Design review of the part built by this model. Coordinates are the model's own, in mm. Coordinates: 2 decimals unless noted, no trailing zeros. Write each loop counter-clockwise with the first axis right and the second up, starting at its lowest first coordinate (ties: lowest second). Pieces come first, ordered by that corner, then holes.
Q1. Take a section at A-A, the plane x = 0. Write out the cut boundary in (y, z).
Q2. Take a section at B-B, the plane z = 0. Write out the cut boundary in (x, y).
Q3. For L1, parallel to X at y = 1.65, z = 0; L2, parallel to X at y = 0.75, z = -13.5; L3, parallel to X at y = 2.6, z = 2, list the stretches that pass through material, from the lowest coordinate up.
Q4. Take a section at D-D, the plane y = 0.65. State how many separate pieces and enclosed holes the cut face has, plus the area to 3 significant figures.
Q5. Take a section at C-C, the plane x = -18.5. Write out the cut boundary in (y, z), plus the area to 3 significant figures.
Q6. For pin 1 Ø1.5 at (x, y) = (9.5, 0.5) entering from -Z; pin 2 Ø1.5 at (y, z) = (2, -13) entering from -X; pin 3 Ø2.5 at (x, z) = (-9.5, 0) entering from -Y, all flat-tipped, find the tip position at first contact; note any pin that passes through.
from build123d import *

# Parameters (mm, degrees)
SKETCH_1_R      = 25
SKETCH_1_R_2    = 5
SKETCH_1_R_3    = 1.5
SKETCH_1_R_4    = 2.5
EXTRUDE_1_DEPTH = 3


with BuildPart() as part:
    # 草圖1 → 填料-伸長1 (new body)
    with BuildSketch(Plane(origin=(0, 0, 0), x_dir=(1, 0, 0), z_dir=(0, 1, 0))):
        with Locations(Location((0, 0, 0), (0, 0, 270))):
            Circle(SKETCH_1_R)
        with Locations(Location((0, 0, 0), (0, 0, 270))):
            Circle(SKETCH_1_R_2, mode=Mode.SUBTRACT)
        with Locations(Location((-9.5, 0, 0), (0, 0, 270))):
            Circle(SKETCH_1_R_3, mode=Mode.SUBTRACT)
        with Locations(Location((9.5, 0, 0), (0, 0, 270))):
            Circle(SKETCH_1_R_3, mode=Mode.SUBTRACT)
        with Locations(Location((0, 19.5, 0), (0, 0, 270))):
            Circle(SKETCH_1_R_4, mode=Mode.SUBTRACT)
        with Locations(Location((19.5, 0, 0), (0, 0, 270))):
            Circle(SKETCH_1_R_4, mode=Mode.SUBTRACT)
        with Locations(Location((0, -19.5, 0), (0, 0, 270))):
            Circle(SKETCH_1_R_4, mode=Mode.SUBTRACT)
        with Locations(Location((-19.5, 0, 0), (0, 0, 270))):
            Circle(SKETCH_1_R_4, mode=Mode.SUBTRACT)
        with Locations(Location((-13.788582233, 13.788582233, 0), (0, 0, 270))):
            Circle(SKETCH_1_R_3, mode=Mode.SUBTRACT)
        with Locations(Location((13.788582233, 13.788582233, 0), (0, 0, 270))):
            Circle(SKETCH_1_R_3, mode=Mode.SUBTRACT)
        with Locations(Location((13.788582233, -13.788582233, 0), (0, 0, 270))):
            Circle(SKETCH_1_R_3, mode=Mode.SUBTRACT)
        with BuildLine():
            ThreePointArc((-20.845079102, -9.72022002), (-16.263455967, -16.263455967), (-9.72022002, -20.845079102))
            ThreePointArc((-9.72022002, -20.845079102), (-5.068978849, -19.152165763), (-6.761892188, -14.500924593))
            ThreePointArc((-6.761892188, -14.500924593), (-11.313708499, -11.313708499), (-14.500924593, -6.761892188))
            ThreePointArc((-14.500924593, -6.761892188), (-19.152165763, -5.068978849), (-20.845079102, -9.72022002))
        make_face(mode=Mode.SUBTRACT)
    extrude(amount=EXTRUDE_1_DEPTH)


solid = part.part
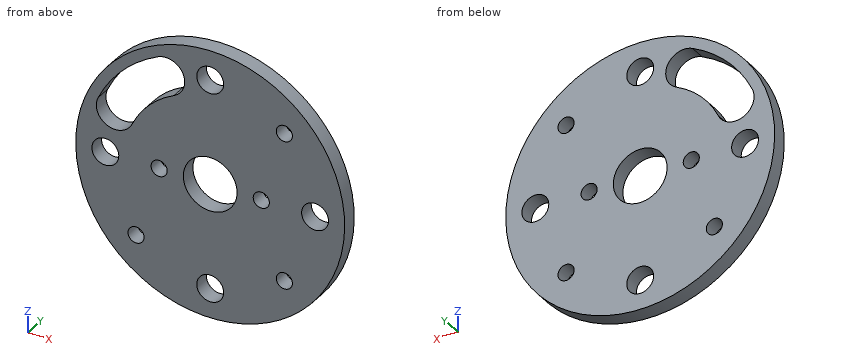
Responses:
1. outline: (0, -25) - (3, -25) - (3, -22) - (0, -22) - close; (0, -17) - (3, -17) - (3, -5) - (0, -5) - close; (0, 5) - (3, 5) - (3, 17) - (0, 17) - close; (0, 22) - (3, 22) - (3, 25) - (0, 25) - close
2. outline: (-25, 0) - (-22, 0) - (-22, 3) - (-25, 3) - close; (-17, 0) - (-11, 0) - (-11, 3) - (-17, 3) - close; (-8, 0) - (-5, 0) - (-5, 3) - (-8, 3) - close; (5, 0) - (8, 0) - (8, 3) - (5, 3) - close; (11, 0) - (17, 0) - (17, 3) - (11, 3) - close; (22, 0) - (25, 0) - (25, 3) - (22, 3) - close
3. L1: x = -25 to -22, -17 to -11, -8 to -5, 5 to 8, 11 to 17, 22 to 25
3. L2: x = -21.04 to -15.26, -12.32 to 12.32, 15.26 to 21.04
3. L3: x = -24.92 to -21, -18 to -4.58, 4.58 to 18, 21 to 24.92
4. separate pieces: 1
4. enclosed holes: 11
4. area: 1,640 mm2
5. outline: (0, -16.82) - (3, -16.82) - (3, -2.29) - (0, -2.29) - close; (0, 2.29) - (3, 2.29) - (3, 4.84) - (0, 4.84) - close; (0, 13.67) - (3, 13.67) - (3, 16.82) - (0, 16.82) - close
5. area: 60.7 mm2
6. pin 1: stops at z = -23.42
6. pin 2: stops at x = -21.79
6. pin 3: passes through
